Model file for the job. Use its own axes, mm. Face numbers are marked on the shaded views. A direction names the side the tool comes from. Give positions to 0.01 mm unless a question says otherwise; leave off trailing zeros. Order: outer loops, then holes, each group sorted by start corner. A loop starts at its lowest first (then second) coordinate and runs counter-clockwise, first axis right, second up. Notation, with made-up numbers: (46, 21) - (80, 21) arc R16 cw to (80, 51) - close; hole circle Ø7 at (69, 4.25). An arc over 180 degrees is marked (long way). Use CSV: the item, a comma, the result in double quotes. Start each with the question number.
(1) Band-saw the part on A-A, the plane z = 8. Give the cut face in (x, y).
(2) Drop flat-ended pins along their axis: pin 1 Ø9.5 at (x, y) = (-2.5, -8) entering from +Z; pin 2 Ø4 at (x, y) = (-6, 11.5) entering from -Z; pin 3 Ø13 at (y, z) = (16.5, 8.5) entering from +X; pin 4 Ø8 at (y, z) = (-13.5, 13.5) entering from -X. Give the stop position or say it passes through.
(3) Band-saw the part on C-C, the plane y = 26. Give the cut face in (x, z).
(4) Pull direction Z, two halves, no side cores. Call the marked faces 1, 2, 3 and 4: +Z half, -Z half, draft (parallel to the pull), parting line (faces both ways), or undercut.
(5) Probe L1, parallel to X at y = 0, z = 31; L2, parallel to Z at x = 1.5, y = -6.5; L3, parallel to Y at x = 0, z = 33. List the from-to ranges inside material, lowest first.
(6) Band-saw the part on D-D, the plane z = 24. Give the cut face in (x, y), then the cut area to 3 significant figures.
(7) Tool access for the marked faces 5, 6, 7 and 8: list every direction of +Z, -Z, +X, -X, +Y, -Y with a clear straight run to the whole face (end or side of a thin tool).
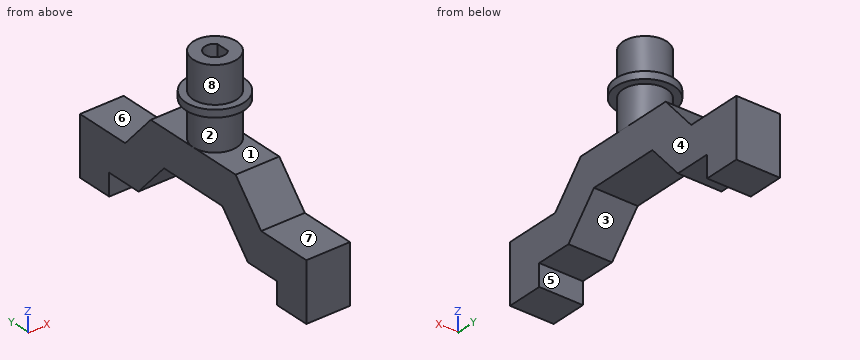
from build123d import *

# Parameters (mm, degrees)
PAD_DEPTH    = 12
SKETCH002_R  = 6
PAD001_DEPTH = 10
SKETCH003_R  = 8
PAD002_DEPTH = 2
SKETCH004_R  = 6
PAD003_DEPTH = 10
POCKET_DEPTH = 21


with BuildPart() as part:
    # Sketch → Pad (new body)
    with BuildSketch(Plane.YZ.offset(-6)):
        Polygon((-38.75, 0), (-38.75, 16), (-23.287682, 16), (-14.537682, 26), (14.537682, 26), (23.287682, 16), (38.75, 16), (38.75, 0), (28.75, 0), (28.75, 6), (18.75, 6), (10, 16), (-10, 16), (-18.75, 6), (-28.75, 6), (-28.75, 0), align=None)
    extrude(amount=PAD_DEPTH)

    # Sketch002 → Pad001 (new body)
    with BuildSketch(Plane(origin=(-6, 0, 26), x_dir=(0, -1, 0), z_dir=(0, 0, 1))):
        with Locations((0, 6)):
            Circle(SKETCH002_R)
    extrude(amount=PAD001_DEPTH)

    # Sketch003 → Pad002 (new body)
    with BuildSketch(Plane(origin=(-6, 0, 36), x_dir=(0, -1, 0), z_dir=(0, 0, 1))):
        with Locations((0, 6)):
            Circle(SKETCH003_R)
    extrude(amount=PAD002_DEPTH)

    # Sketch004 → Pad003 (new body)
    with BuildSketch(Plane(origin=(-6, 0, 38), x_dir=(0, -1, 0), z_dir=(0, 0, 1))):
        with Locations((0, 6)):
            Circle(SKETCH004_R)
    extrude(amount=PAD003_DEPTH)

    # Sketch005 → Pocket (cut)
    with BuildSketch(Plane(origin=(-6, 0, 48), x_dir=(0, -1, 0), z_dir=(0, 0, 1))):
        with BuildLine():
            Line((-1.821648, 8.1), (1.821648, 8.1))
            ThreePointArc((-1.821648, 8.1), (0, 3.22), (1.821648, 8.1))
        make_face()
    extrude(amount=-POCKET_DEPTH, mode=Mode.SUBTRACT)


solid = part.part
Answer block:
1,outline,"(-6, -38.75) - (6, -38.75) - (6, -17) - (-6, -17) - close; (-6, 17) - (6, 17) - (6, 38.75) - (-6, 38.75) - close"
2,pin 1,"stops at z = 48"
2,pin 2,"stops at z = 12"
2,pin 3,"stops at x = 6"
2,pin 4,"stops at x = -6"
3,outline,"(-6, 6) - (6, 6) - (6, 16) - (-6, 16) - close"
4,face 1,"undercut"
4,face 2,"undercut"
4,face 3,"-Z half"
4,face 4,"draft"
5,L1,"x = -6 to -2.78, 2.1 to 6"
5,L2,"z = 16 to 26, 36 to 38"
5,L3,"y = -6 to -2.78, 2.78 to 6"
6,outline,"(-6, -16.29) - (6, -16.29) - (6, 16.29) - (-6, 16.29) - close"
6,area,"391 mm2"
7,face 5,"-Z, +X, -X"
7,face 6,"+Z, +X, -X, +Y"
7,face 7,"+Z, +X, -X, -Y"
7,face 8,"+Z"
